CAD build for the part. Positions are in the model's coordinates, mm. Face numbers are marked on the shaded views. A direction names the side the tool comes from. Coordinates: 2 decimals unless noted, no trailing zeros.
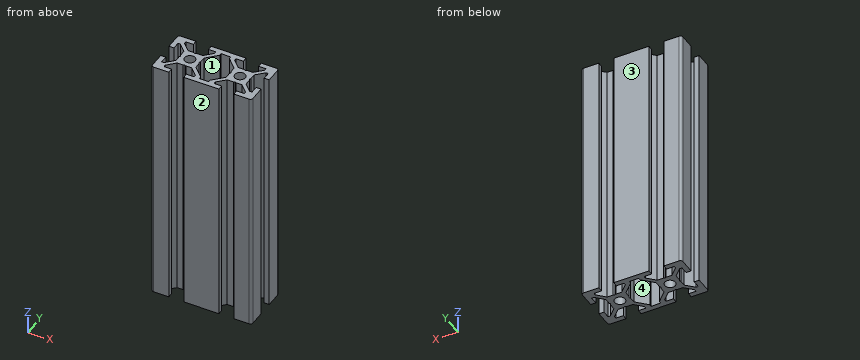
```python
from build123d import *

# Parameters (mm, degrees)
F0_R     = 2.1
F1_DEPTH = 100


with BuildPart() as f1:
    # F0 (on Top) → F1 (new body)
    with BuildSketch(Plane.XY):
        with BuildLine():
            Line((14.135135, -0.519615), (13.835135, 0))
            Line((13.835135, 0), (14.135135, 0.519615))
            Line((14.135135, 0.519615), (14.135135, 2.93934))
            Line((14.135135, 2.93934), (17.195795, 6))
            Line((17.195795, 6), (18.135135, 6))
            Line((18.135135, 6), (18.135135, 3))
            Line((18.135135, 3), (20.135135, 3))
            Line((20.135135, 3), (20.135135, 9))
            ThreePointArc((20.135135, 9), (19.842242, 9.707107), (19.135135, 10))
            Line((19.135135, 10), (13.135135, 10))
            Line((13.135135, 10), (13.135135, 8))
            Line((13.135135, 8), (16.135135, 8))
            Line((16.135135, 8), (16.135135, 7.06066))
            Line((16.135135, 7.06066), (13.074475, 4))
            Line((13.074475, 4), (10.65475, 4))
            Line((10.65475, 4), (10.135135, 3.7))
            Line((10.135135, 3.7), (9.61552, 4))
            Line((9.61552, 4), (7.195795, 4))
            Line((7.195795, 4), (4.135135, 7.06066))
            Line((4.135135, 7.06066), (4.135135, 8))
            Line((4.135135, 8), (7.135135, 8))
            Line((7.135135, 8), (7.135135, 10))
            Line((7.135135, 10), (-6.864865, 10))
            Line((-6.864865, 10), (-6.864865, 8))
            Line((-6.864865, 8), (-3.864865, 8))
            Line((-3.864865, 8), (-3.864865, 7.06066))
            Line((-3.864865, 7.06066), (-6.925525, 4))
            Line((-6.925525, 4), (-9.34525, 4))
            Line((-9.34525, 4), (-9.864865, 3.7))
            Line((-9.864865, 3.7), (-10.38448, 4))
            Line((-10.38448, 4), (-12.804205, 4))
            Line((-12.804205, 4), (-15.864865, 7.06066))
            Line((-15.864865, 7.06066), (-15.864865, 8))
            Line((-15.864865, 8), (-12.864865, 8))
            Line((-12.864865, 8), (-12.864865, 10))
            Line((-12.864865, 10), (-18.864865, 10))
            ThreePointArc((-18.864865, 10), (-19.571972, 9.707107), (-19.864865, 9))
            Line((-19.864865, 9), (-19.864865, 3))
            Line((-19.864865, 3), (-17.864865, 3))
            Line((-17.864865, 3), (-17.864865, 6))
            Line((-17.864865, 6), (-16.925525, 6))
            Line((-16.925525, 6), (-13.864865, 2.93934))
            Line((-13.864865, 2.93934), (-13.864865, 0.519615))
            Line((-13.864865, 0.519615), (-13.564865, 0))
            Line((-13.564865, 0), (-13.864865, -0.519615))
            Line((-13.864865, -0.519615), (-13.864865, -2.93934))
            Line((-13.864865, -2.93934), (-16.925525, -6))
            Line((-16.925525, -6), (-17.864865, -6))
            Line((-17.864865, -6), (-17.864865, -3))
            Line((-17.864865, -3), (-19.864865, -3))
            Line((-19.864865, -3), (-19.864865, -9))
            ThreePointArc((-19.864865, -9), (-19.571972, -9.707107), (-18.864865, -10))
            Line((-18.864865, -10), (-12.864865, -10))
            Line((-12.864865, -10), (-12.864865, -8))
            Line((-12.864865, -8), (-15.864865, -8))
            Line((-15.864865, -8), (-15.864865, -7.06066))
            Line((-15.864865, -7.06066), (-12.804205, -4))
            Line((-12.804205, -4), (-10.38448, -4))
            Line((-10.38448, -4), (-9.864865, -3.7))
            Line((-9.864865, -3.7), (-9.34525, -4))
            Line((-9.34525, -4), (-6.925525, -4))
            Line((-6.925525, -4), (-3.864865, -7.06066))
            Line((-3.864865, -7.06066), (-3.864865, -8))
            Line((-3.864865, -8), (-6.864865, -8))
            Line((-6.864865, -8), (-6.864865, -10))
            Line((-6.864865, -10), (7.135135, -10))
            Line((7.135135, -10), (7.135135, -8))
            Line((7.135135, -8), (4.135135, -8))
            Line((4.135135, -8), (4.135135, -7.06066))
            Line((4.135135, -7.06066), (7.195795, -4))
            Line((7.195795, -4), (9.61552, -4))
            Line((9.61552, -4), (10.135135, -3.7))
            Line((10.135135, -3.7), (10.65475, -4))
            Line((10.65475, -4), (13.074475, -4))
            Line((13.074475, -4), (16.135135, -7.06066))
            Line((16.135135, -7.06066), (16.135135, -8))
            Line((16.135135, -8), (13.135135, -8))
            Line((13.135135, -8), (13.135135, -10))
            Line((13.135135, -10), (19.135135, -10))
            ThreePointArc((19.135135, -10), (19.842242, -9.707107), (20.135135, -9))
            Line((20.135135, -9), (20.135135, -3))
            Line((20.135135, -3), (18.135135, -3))
            Line((18.135135, -3), (18.135135, -6))
            Line((18.135135, -6), (17.195795, -6))
            Line((17.195795, -6), (14.135135, -2.93934))
            Line((14.135135, -2.93934), (14.135135, -0.519615))
        make_face()
        with Locations((-9.864865, 0)):
            Circle(F0_R, mode=Mode.SUBTRACT)
        Polygon((6.435135, 0), (6.135135, -0.519615), (6.135135, -2.93934), (3.074475, -6), (2.013815, -7.06066), (2.013815, -8), (-1.743545, -8), (-1.743545, -7.06066), (-2.804205, -6), (-5.864865, -2.93934), (-5.864865, -0.519615), (-6.164865, 0), (-5.864865, 0.519615), (-5.864865, 2.93934), (-2.804205, 6), (-1.743545, 7.06066), (-1.743545, 8), (2.013815, 8), (2.013815, 7.06066), (3.074475, 6), (6.135135, 2.93934), (6.135135, 0.519615), align=None, mode=Mode.SUBTRACT)
        with Locations((10.135135, 0)):
            Circle(F0_R, mode=Mode.SUBTRACT)
    extrude(amount=F1_DEPTH)


solid = f1.part
```
Item 1: Which spindle directions (+Z, -Z, +X, -X, +Y, -Y) get a long thin tool onto all of the face, cutting with end or side? Do the marked faces 1 and 2. Say none if no direction does.
Item 2: Two-plate mould, pull along X, no slides. Class the marked faces 3 and 4: +X half, -X half, draft (parallel to the pull), parting line (faces both ways), or undercut.
Item 3: Flat gauge pins, fed straight in: pin 1 Ø6 at (x, y) = (11, 4.5) entering from -Z; pin 2 Ø5 at (x, z) = (-9.5, 75) entering from -Y; pin 3 Ø0.6 at (y, z) = (-9.5, 69.5) entering from +X; pin 4 Ø0.7 at (x, z) = (-7.5, 65.5) entering from +Y. Where does each tip first touch, or does it go through?
Item 4: Saw through at A-A, the plane z = 31.5. State how many separate pieces and enclosed holes the cut face has, and give its area (3 significant figures).
Item 5: Wall check: line 1 along X through (y, z) = (-7.25, 5); line 2 along X through (y, z) = (-8.5, 37); line 3 along Y through (x, z) = (-4.5, 14). Give the ranges that are in metal, low to high.
Working result:
1. face 1: +Z, -Z
1. face 2: +Z, -Z, +X, -X, -Y
2. face 3: draft
2. face 4: undercut
3. pin 1: stops at z = 0
3. pin 2: stops at y = -4
3. pin 3: stops at x = 20.11
3. pin 4: stops at y = 4
4. separate pieces: 1
4. enclosed holes: 3
4. area: 324 mm2
5. line 1: x = -19.86 to -15.86, -3.86 to -1.74, 2.01 to 4.14, 16.14 to 20.14
5. line 2: x = -19.86 to -12.86, -6.86 to 7.14, 13.14 to 20.14
5. line 3: y = -10 to -8, -6.43 to -4.3, 4.3 to 6.43, 8 to 10
